from build123d import *

# Parameters (mm, degrees)
SKETCH_1_W                       = 71
SKETCH_1_H                       = 32
EXTRUDE_1_DEPTH                  = 3.15
SKETCH_2_W                       = 3.15
SKETCH_2_H                       = 32
EXTRUDE_2_DEPTH                  = 14
FILLET_1_R                       = 2
SKETCH_3_R                       = 1.7
SKETCH_3_R_2                     = 1.2
CUT_EXTRUDE_1_DEPTH              = 43.548472358
CUT_EXTRUDE_2_DEPTH              = 75.773808917
SKETCH_7_W                       = 32
SKETCH_7_H                       = 3.15
CUT_EXTRUDE_3_DEPTH              = 15
HOLE_WIZARD_M2_2_D               = 1.6
HOLE_WIZARD_M2_2_DEPTH           = 4
HOLE_WIZARD_M2_2_TIP             = 0.480688495
HOLE_WIZARD_M2_2_ON_FACE_2_D     = 1.6
HOLE_WIZARD_M2_2_ON_FACE_2_DEPTH = 4
HOLE_WIZARD_M2_2_ON_FACE_2_TIP   = 0.480688495


with BuildPart() as part:
    # 草图1 → 凸台-拉伸1 (new body)
    with BuildSketch(Plane(origin=(0, 0, 0), x_dir=(1, 0, 0), z_dir=(0, 1, 0))):
        Rectangle(SKETCH_1_W, SKETCH_1_H)
    extrude(amount=EXTRUDE_1_DEPTH)

    # 草图2 → 凸台-拉伸2 (add)
    with BuildSketch(Plane(origin=(0, 3.15, 0), x_dir=(1, 0, 0), z_dir=(0, 1, 0))):
        with Locations((33.925, 0)):
            Rectangle(SKETCH_2_W, SKETCH_2_H)
    extrude(amount=EXTRUDE_2_DEPTH)

    # 圆角1
    fillet_1_edges = [part.edges().sort_by_distance(p)[0] for p in [
        (32.35, 3.15, 0),
        (35.5, 0, 0),
    ]]
    fillet(fillet_1_edges, radius=FILLET_1_R)

    # 草图3 → 切除-拉伸1 (cut, through all)
    with BuildSketch(Plane.XZ):
        with Locations(Location((-2, -10.7, 0), (0, 0, 270))):
            Circle(SKETCH_3_R)
        with Locations(Location((8.5, 2.3, 0), (0, 0, 270))):
            Circle(SKETCH_3_R_2)
    extrude(amount=-CUT_EXTRUDE_1_DEPTH, mode=Mode.SUBTRACT)

    # 草图5 → M2x0.4 螺纹孔1 (revolve, cut)
    with BuildSketch(Plane(origin=(19.5, 1.575, 16), x_dir=(0, -1, 0), z_dir=(1, 0, 0))):
        Polygon((0, 0), (0, 5.680688495), (0.8, 5.2), (0.8, 0), align=None)
    m2x0_4_1 = revolve(axis=Axis((19.5, 1.575, 22.35), (0, 0, -1)), mode=Mode.SUBTRACT)

    # 镜向1: M2x0.4 螺纹孔1 across plane
    add(m2x0_4_1.mirror(Plane.XY), mode=Mode.SUBTRACT)

    # 草图6 → 切除-拉伸2 (cut, through all)
    with BuildSketch(Plane(origin=(35.5, 0, 0), x_dir=(0, 0, -1), z_dir=(1, 0, 0))):
        with BuildLine():
            Line((-13, 13.85), (13, 13.85))
            ThreePointArc((13, 13.85), (14.7, 12.15), (13, 10.45))
            Line((13, 10.45), (-13, 10.45))
            ThreePointArc((-13, 10.45), (-14.7, 12.15), (-13, 13.85))
        make_face()
    extrude(amount=-CUT_EXTRUDE_2_DEPTH, mode=Mode.SUBTRACT)

    # 草图7 → 切除-拉伸3 (cut)
    with BuildSketch(Plane.ZY.offset(35.5)):
        with Locations((0, 1.575)):
            Rectangle(SKETCH_7_W, SKETCH_7_H)
    extrude(amount=-CUT_EXTRUDE_3_DEPTH, mode=Mode.SUBTRACT)

    # M2 螺纹孔2
    with Locations(Plane(origin=(-10.5, 1.575, 16), x_dir=(1, 0, 0), z_dir=(0, 0, 1))):
        with Locations((0, 0)):
            Hole(HOLE_WIZARD_M2_2_D / 2, depth=HOLE_WIZARD_M2_2_DEPTH)
            with Locations((0, 0, -(HOLE_WIZARD_M2_2_DEPTH + HOLE_WIZARD_M2_2_TIP / 2))):  # 118° drill point
                Cone(0, HOLE_WIZARD_M2_2_D / 2, HOLE_WIZARD_M2_2_TIP, mode=Mode.SUBTRACT)

    # M2 螺纹孔2 on face 2
    with Locations(Plane(origin=(-10.5, 1.575, -16), x_dir=(-1, 0, 0), z_dir=(0, 0, -1))):
        with Locations((0, 0)):
            Hole(HOLE_WIZARD_M2_2_ON_FACE_2_D / 2, depth=HOLE_WIZARD_M2_2_ON_FACE_2_DEPTH)
            with Locations((0, 0, -(HOLE_WIZARD_M2_2_ON_FACE_2_DEPTH + HOLE_WIZARD_M2_2_ON_FACE_2_TIP / 2))):  # 118° drill point
                Cone(0, HOLE_WIZARD_M2_2_ON_FACE_2_D / 2, HOLE_WIZARD_M2_2_ON_FACE_2_TIP, mode=Mode.SUBTRACT)


solid = part.part
Work out the finished part from the listing and answer in its coordinate system (mm). A direction names the side the tool comes from. Round coordinates to 2 decimals unless told otherwise and drop trailing zeros. Write each loop counter-clockwise with the first axis right and the second up, starting at its lowest first coordinate (ties: lowest second). Pieces come first, ordered by that corner, then holes.
1) A tool of negligible diameter and unlimited length cuts with its end or side. For faces 1 (the flat face through (34, 10.45, 0)), 2 (the flat face through (5, 3.15, 0)), 3 (the cylindrical face through (20.21, 1.21, -13.44)), from which of +Z, -Z, +X, -X, +Y, -Y can it reach the whole face along a straight path? Write none if from no direction.
2) Given pin 1 Ø3.5 at (x, z) = (34.5, -6) entering from -Y; pin 2 Ø1.5 at (y, z) = (9, -1) entering from -X; pin 3 Ø1 at (x, y) = (-10.5, 1.575) entering from +Z; pin 4 Ø10 at (x, z) = (-12, -0.5) entering from +Y, each flat-ended and moving along its own axis, determine where each tip first touches the part or whether it passes through.
3) A cutting plane is placed at D-D (x = 26.5). Give the vertices of the cut face in (y, z), plus the area to 3 significant figures.
4) A cutting plane is placed at B-B (y = 12.15). Give the vertices of the cut face in (x, z), plus the area to 3 significant figures.
5) Straight lines are drawn through the part: line 1 (Y direction, x = 19.5, z = 14.3) (3 decimals); line 2 (Y direction, x = 16.5, z = 10). For each, find the intervals that lie inside material, in ascending order.
6) A cutting plane is placed at C-C (z = 8). Give the vertices of the cut face in (x, y), plus the area to 3 significant figures.
7) The mould has two halves that part along X. Classify faces 4 (the cylindrical face through (-10.131, 0.865, -13.972)), 5 (the cylindrical face through (34.93, 0.6, -0.22)), 6 (the cylindrical face through (33.9, 12.1, 14.7)), 7 (the flat face through (32.35, 10, 0)): pulls with the +X half, pulls with the -X half, needs draft (parallel to the pull), parting line crosses it, or undercut.
8) A cutting plane is placed at A-A (x = 8.5). Give the vertices of the cut face in (y, z), plus the area to 3 significant figures.
Completed:
1. face 1: +X, -X
1. face 2: +Z, -Z, -X, +Y
1. face 3: -Z
2. pin 1: stops at y = 0
2. pin 2: stops at x = 32.35
2. pin 3: stops at z = 11.82
2. pin 4: stops at y = 3.15
3. outline: (0, -16) - (3.15, -16) - (3.15, 16) - (0, 16) - close
3. area: 101 mm2
4. outline: (32.35, -16) - (35.5, -16) - (35.5, -14.7) - (32.35, -14.7) - close; (32.35, 14.7) - (35.5, 14.7) - (35.5, 16) - (32.35, 16) - close
4. area: 8.19 mm2
5. line 1: y = 0 to 0.775, 2.375 to 3.15
5. line 2: y = 0 to 3.15
6. outline: (-20.5, 0) - (33.5, 0) arc R2 ccw to (35.5, 2) - (35.5, 10.45) - (32.35, 10.45) - (32.35, 5.15) arc R2 cw to (30.35, 3.15) - (-20.5, 3.15) - close; (32.35, 13.85) - (35.5, 13.85) - (35.5, 17.15) - (32.35, 17.15) - close
6. area: 210 mm2
7. face 4: undercut
7. face 5: pulls with the +X half
7. face 6: needs draft
7. face 7: pulls with the -X half
8. outline: (0, -16) - (3.15, -16) - (3.15, 1.1) - (0, 1.1) - close; (0, 3.5) - (3.15, 3.5) - (3.15, 16) - (0, 16) - close
8. area: 93.2 mm2
